Source: three-view drawing plus pictorial views. Frame: mm from the lowest corner of the part. A direction names the side the tool comes from. Give positions to 0.01 mm unless a question says otherwise; leave off trailing zeros. Order: outer loops, then holes, each group sorted by start corner. A loop starts at its lowest first (then second) coordinate and runs counter-clockwise, first axis right, second up. Notation, with made-up numbers: (68, 21) - (88, 21) arc R10 ccw to (88, 38) - close; hole circle Ø7 at (3.25, 26). An arc over 180 degrees is marked (long way). Use CSV: the item, a comma, the result in double quotes.
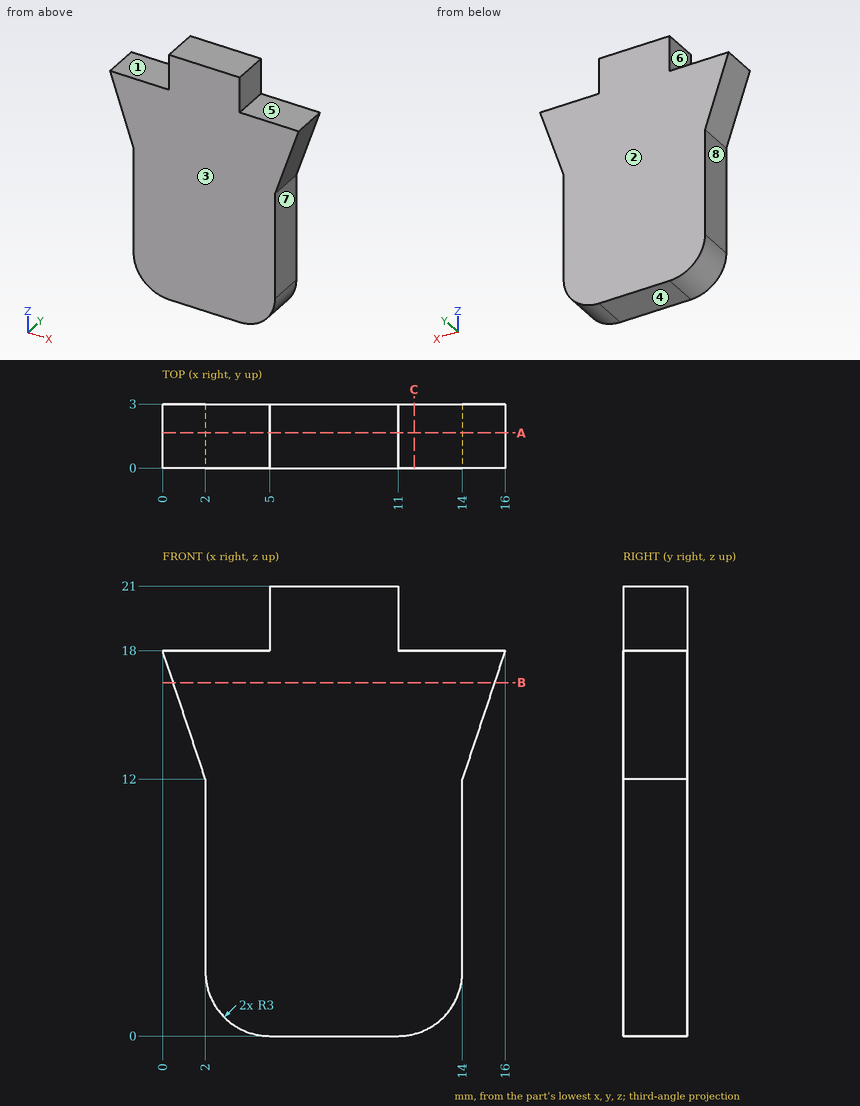
Item 1: First-contact query: pin 1 (0.9 mm diameter, centred on y = 1, z = 6.5, fed in from +X); pin 2 (1.5 mm diameter, centred on y = 1.5, z = 19, fed in from +X); pin 3 (1.5 mm diameter, centred on y = 1, z = 20, fed in from -X). Flat tips, straight axial feed; report the tip coordinate or a pass-through.
Filled in:
pin 1,"stops at x = 14"
pin 2,"stops at x = 11"
pin 3,"stops at x = 5"
Item 2: Section B-B on z = 16.5. Return the cut outline in (x, y), then the cut area to 3 significant figures.
Filled in:
outline,"(0.5, 0) - (15.5, 0) - (15.5, 3) - (0.5, 3) - close"
area,"45.0 mm2"
Item 3: Mould query, pull axis Y, two halves, no side actions, for the marked faces 1, 2 and 3. Classes: released by +Y, released by -Y, zero draft, split by the parting line, or undercut.
Filled in:
face 1,"zero draft"
face 2,"released by +Y"
face 3,"released by -Y"
Item 4: Section C-C on x = 11.75. Return the cut outline in (y, z).
Filled in:
outline,"(0, 0.1) - (3, 0.1) - (3, 18) - (0, 18) - close"
Item 5: Material intervals for line 1 (X direction, y = 0.7, z = 4.5); line 2 (X direction, y = 0.7, z = 13.5); line 3 (Z direction, x = 11.75, y = 1.85), sorted ascending. Write a range as from..to.
Filled in:
line 1,"x = 2..14"
line 2,"x = 1.5..14.5"
line 3,"z = 0.1..18"
Item 6: Section A-A on y = 1.65. Return the cut outline in (x, z).
Filled in:
outline,"(0, 18) - (2, 12) - (2, 3) arc R3 ccw to (5, 0) - (11, 0) arc R3 ccw to (14, 3) - (14, 12) - (16, 18) - (11, 18) - (11, 21) - (5, 21) - (5, 18) - close"
Item 7: Set-up query: the marked faces 4, 5, 6, 7 and 8. Return all of +Z, -Z, +X, -X, +Y, -Y with unobstructed straight access to the full face (end or side cutting, diameter ignored); none if empty.
Filled in:
face 4,"-Z, +X, -X, +Y, -Y"
face 5,"+Z, +X, +Y, -Y"
face 6,"+Z, -X, +Y, -Y"
face 7,"-Z, +X, +Y, -Y"
face 8,"-Z, -X, +Y, -Y"
